Geometry: final body of the model. Coordinates: model frame, mm. A direction names the side the tool comes from. Give positions to 0.01 mm unless a question says otherwise; leave off trailing zeros. Write each loop counter-clockwise with the first axis right and the second up, starting at its lowest first coordinate (ties: lowest second). Pieces come first, ordered by that corner, then holes.
Q1. Mould query, pull axis X, two halves, no side actions, for faces 4 (the flat face through (-30, -45, 5)), 5 (the flat face through (-49, 55, 7.8)), 6 (the flat face through (-60, 1, 2)). Classes: +X half, -X half, draft (parallel to the pull), parting line (faces both ways), or undercut.
Q2. Reachability of faces 1 (the flat face through (45, -55, 4.6)), 2 (the flat face through (-45, -42, 3.8)), 3 (the flat face through (1, -60, 2)) from +Z, -Z, +X, -X, +Y, -Y: full face, straight path, thin tool, end or side. Return the list, or none.
Q3. Line query: line 1 (X direction, y = 35, z = 4.5); line 2 (X direction, y = 36, z = 5); line 3 (Y direction, x = -51, z = 7). Output: solid intervals per line, ascending.
Q4. Pin query (flat end, axial travel): pin 1 Ø6 at (x, y) = (-6.5, 4.5) entering from -Z; pin 2 Ø1 at (x, y) = (-2.5, -4.5) entering from +Z; pin 3 Ø1.5 at (x, y) = (47, 43) entering from +Z. Return the tip coordinate at first contact, or that it passes through.
Q5. Section A-A (x = -46). Return the cut outline in (y, z), plus the area to 3 significant figures.
Q6. Section C-C (x = -26.5). Return the cut outline in (y, z).
from build123d import *

# Parameters (mm, degrees)
SKETCH_W           = 120
SKETCH_H           = 120
PAD_DEPTH          = 3
SKETCH001_W        = 30
SKETCH001_H        = 30
PAD001_DEPTH       = 4.8
SKETCH002_W        = 27
SKETCH002_H        = 1.6
POCKET_DEPTH       = 369.770569
SKETCH003_W        = 20
SKETCH003_H        = 24
POCKET001_DEPTH    = 4
POLARPATTERN_COUNT = 2


with BuildPart() as part:
    # Sketch → Pad (new body)
    with BuildSketch(Plane.XY):
        Rectangle(SKETCH_W, SKETCH_H)
    extrude(amount=PAD_DEPTH)

    # Sketch001 (on Face6 of Pad) → Pad001 (join)
    with BuildSketch(Plane.XY.offset(3)):
        with Locations((-45, 45)):
            Rectangle(SKETCH001_W, SKETCH001_H)
    pad001 = extrude(amount=PAD001_DEPTH)

    # Sketch002 (on Face7 of Pad001) → Pocket (cut, through all)
    with BuildSketch(Plane.XZ.offset(-30)):
        with Locations((-45, 5.4)):
            Rectangle(SKETCH002_W, SKETCH002_H)
    pocket = extrude(amount=-POCKET_DEPTH, mode=Mode.SUBTRACT)

    # Sketch003 (on Face7 of Pocket) → Pocket001 (cut)
    with BuildSketch(Plane.XY.offset(7.8)):
        with Locations((-45, 42)):
            Rectangle(SKETCH003_W, SKETCH003_H)
    pocket001 = extrude(amount=-POCKET001_DEPTH, mode=Mode.SUBTRACT)

    # Mirrored: Pad001, Pocket, Pocket001 across Sketch001 V_Axis
    add(pad001.mirror(Plane(origin=(0, 0, 3), x_dir=(0, 0, 1), z_dir=(1, 0, 0))))
    add(pocket.mirror(Plane(origin=(0, 0, 3), x_dir=(0, 0, 1), z_dir=(1, 0, 0))), mode=Mode.SUBTRACT)
    add(pocket001.mirror(Plane(origin=(0, 0, 3), x_dir=(0, 0, 1), z_dir=(1, 0, 0))), mode=Mode.SUBTRACT)

    # Mirrored001: Pad001, Pocket, Pocket001 across Sketch001 H_Axis
    add(pad001.mirror(Plane(origin=(0, 0, 3), x_dir=(0, 0, 1), z_dir=(0, 1, 0))))
    add(pocket.mirror(Plane(origin=(0, 0, 3), x_dir=(0, 0, 1), z_dir=(0, 1, 0))), mode=Mode.SUBTRACT)
    add(pocket001.mirror(Plane(origin=(0, 0, 3), x_dir=(0, 0, 1), z_dir=(0, 1, 0))), mode=Mode.SUBTRACT)

    # PolarPattern: Pad001, Pocket, Pocket001 ×2 about axis
    polarpattern_axis = Axis((0, 0, 3), (0, 0, 1))
    for i in range(1, POLARPATTERN_COUNT):
        add(pad001.rotate(polarpattern_axis, i * 360 / POLARPATTERN_COUNT))
        add(pocket.rotate(polarpattern_axis, i * 360 / POLARPATTERN_COUNT), mode=Mode.SUBTRACT)
        add(pocket001.rotate(polarpattern_axis, i * 360 / POLARPATTERN_COUNT), mode=Mode.SUBTRACT)


solid = part.part
Computed:
1. face 4: undercut
1. face 5: draft
1. face 6: -X half
2. face 1: +Y, -Y
2. face 2: +Z
2. face 3: +Z, -Z, +X, -X, -Y
3. line 1: x = -60 to -55, -35 to -30, 30 to 35, 55 to 60
3. line 2: x = -60 to -58.5, -31.5 to -30, 30 to 31.5, 58.5 to 60
3. line 3: y = -60 to -54, 54 to 60
4. pin 1: stops at z = 0
4. pin 2: stops at z = 3
4. pin 3: stops at z = 3.8
5. outline: (-60, 0) - (60, 0) - (60, 4.6) - (54, 4.6) - (54, 3.8) - (30, 3.8) - (30, 3) - (-30, 3) - (-30, 3.8) - (-54, 3.8) - (-54, 4.6) - (-60, 4.6) - close; (-60, 6.2) - (-54, 6.2) - (-54, 7.8) - (-60, 7.8) - close; (54, 6.2) - (60, 6.2) - (60, 7.8) - (54, 7.8) - close
5. area: 437 mm2
6. outline: (-60, 0) - (60, 0) - (60, 3) - (-60, 3) - close
